Build history of the part. All positions in model axes, mm. Round coordinates to 2 decimals unless told otherwise and drop trailing zeros. Write each loop counter-clockwise with the first axis right and the second up, starting at its lowest first coordinate (ties: lowest second). Pieces come first, ordered by that corner, then holes. Notation, with made-up numbers: (-27, 58) -> (-7, 58) arc R8 cw to (-7, 70) -> close; hole circle Ø4 at (55.5, 77.25). An arc over 180 degrees is marked (long way). Answer as CSV lines item,"result".
from build123d import *

# Parameters (mm, degrees)
SKETCH_2_R          = 1.6
EXTRUDE_1_DEPTH     = 10
SKETCH_3_W          = 8
SKETCH_3_H          = 8
CUT_EXTRUDE_1_DEPTH = 140.947387002
SKETCH_4_R          = 1.6
CUT_EXTRUDE_2_DEPTH = 10


with BuildPart() as part:
    # ｽｹｯﾁ2 → ﾎﾞｽ - 押し出し1 (new body)
    with BuildSketch(Plane.XY):
        Polygon((83.071643169, 8.195972832), (-3.936021884, 91.354077293), (-10.845357286, 84.124894469), (77.150331852, 0.022479987), (84.059667254, 7.25166281), align=None)
        with Locations((-3.776098173, 84.28481818)):
            Circle(SKETCH_2_R, mode=Mode.SUBTRACT)
        with Locations((76.990408141, 7.0917391)):
            Circle(SKETCH_2_R, mode=Mode.SUBTRACT)
    extrude(amount=EXTRUDE_1_DEPTH)

    # ｽｹｯﾁ3 → ｶｯﾄ - 押し出し1 (cut, through all)
    with BuildSketch(Plane(origin=(40.308371471, -38.524970914, 0), x_dir=(0, 0, -1), z_dir=(0.7229182823698357, -0.690933540230496, 0))):
        with Locations((-5, 58.32200311)):
            Rectangle(SKETCH_3_W, SKETCH_3_H)
    extrude(amount=-CUT_EXTRUDE_1_DEPTH, mode=Mode.SUBTRACT)

    # ｽｹｯﾁ4 → ｶｯﾄ - 押し出し2 (cut)
    with BuildSketch(Plane.XY.offset(10)):
        with Locations((50.342602349, 32.560541375)):
            Circle(SKETCH_4_R)
        with Locations((22.871707619, 58.816015904)):
            Circle(SKETCH_4_R)
        with Locations((36.607154984, 45.68827864)):
            Circle(SKETCH_4_R)
    extrude(amount=-CUT_EXTRUDE_2_DEPTH, mode=Mode.SUBTRACT)


solid = part.part
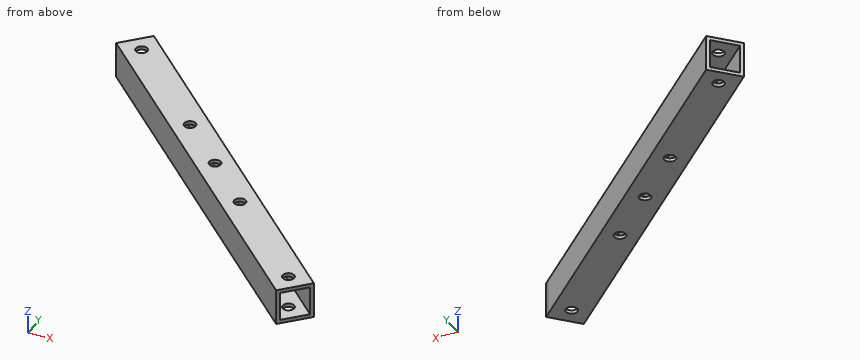
1. Probe line 1 along Z through (x, y) = (-2.5, 82); line 2 along Y through (x, z) = (69, 7); line 3 along Y through (x, z) = (67, 3.5). List the from-to ranges inside material, lowest first.
Results found:
line 1,"z = 0 to 1, 9 to 10"
line 2,"y = 7.81 to 9.2, 20.26 to 21.65"
line 3,"y = 9.72 to 11.11, 22.17 to 23.56"
2. Cut at C-C, the plane y = 41.5. Write the cut outline in (x, z), then the cut area to 3 significant figures.
Results found:
outline,"(33.75, 0) -> (48.23, 0) -> (48.23, 10) -> (33.75, 10) -> close; hole (35.2, 1) -> (46.78, 1) -> (46.78, 9) -> (35.2, 9) -> close"
area,"52.1 mm2"
3. Cut at A-A, the plane z = 5.75. Write the cut outline in (x, y).
Results found:
outline,"(-10.85, 84.12) -> (77.15, 0.02) -> (77.84, 0.75) -> (-10.15, 84.85) -> close; (-4.63, 90.63) -> (83.37, 6.53) -> (84.06, 7.25) -> (-3.94, 91.35) -> close"
4. Drop flat-ended pins along their axis: pin 1 Ø2 at (y, z) = (43, 5) entering from -X; pin 2 Ø2.5 at (x, y) = (36.61, 45.69) entering from +Z; pin 3 Ø3 at (x, z) = (5, 3.5) entering from +Y; pin 4 Ø6 at (y, z) = (19.5, 2) entering from -X. Give the stop position or say it passes through.
Results found:
pin 1,"stops at x = 31.14"
pin 2,"passes through"
pin 3,"stops at y = 84.25"
pin 4,"stops at x = 53.63"
5. Cut at D-D, the plane x = 53.5. Write the cut outline in (y, z).
Results found:
outline,"(22.63, 0) -> (36.46, 0) -> (36.46, 10) -> (22.63, 10) -> close; hole (24.01, 1) -> (35.08, 1) -> (35.08, 9) -> (24.01, 9) -> close"
6. Cut at B-B, the plane x = 36.5. Write the cut outline in (y, z), then the cut area to 3 significant figures.
Results found:
outline,"(38.87, 0) -> (44.09, 0) -> (44.09, 1) -> (40.26, 1) -> (40.26, 9) -> (44.09, 9) -> (44.09, 10) -> (38.87, 10) -> close; (47.28, 0) -> (52.71, 0) -> (52.71, 10) -> (47.28, 10) -> (47.28, 9) -> (51.32, 9) -> (51.32, 1) -> (47.28, 1) -> close"
area,"43.4 mm2"
